```python
from build123d import *

# Parameters (mm, degrees)
BOSS_EXTRUDE1_DEPTH = 3.175
SKETCH2_W           = 25.4
SKETCH2_H           = 17.4625
BOSS_EXTRUDE2_DEPTH = 3.175
SKETCH4_W           = 2.238000096
SKETCH4_H           = 9.5
CUT_EXTRUDE1_DEPTH  = 3.175
SKETCH5_W           = 8.68426
SKETCH5_H           = 7.9625
BOSS_EXTRUDE3_DEPTH = 3.175
CUT_EXTRUDE2_DEPTH  = 3.175


with BuildPart() as part:
    # Sketch1 → Boss-Extrude1 (new body)
    with BuildSketch(Plane.XY):
        Polygon((-12.7, 19.05), (-6.35, 19.05), (-6.35, 15.875), (6.35, 15.875), (6.35, 19.05), (12.7, 19.05), (12.7, -19.05), (6.35, -19.05), (6.35, -15.875), (-6.35, -15.875), (-6.35, -19.05), (-12.7, -19.05), align=None)
    extrude(amount=BOSS_EXTRUDE1_DEPTH)

    # Sketch2 → Boss-Extrude2 (add)
    with BuildSketch(Plane(origin=(0, 0, 0), x_dir=(-1, 0, 0), z_dir=(0, 0, -1))):
        with Locations((0, -27.78125)):
            Rectangle(SKETCH2_W, SKETCH2_H)
    extrude(amount=-BOSS_EXTRUDE2_DEPTH)

    # Sketch4 → Cut-Extrude1 (cut)
    with BuildSketch(Plane(origin=(0, 0, 0), x_dir=(-1, 0, 0), z_dir=(0, 0, -1))):
        with Locations((-11.580999952, -23.8)):
            Rectangle(SKETCH4_W, SKETCH4_H)
    cut_extrude1 = extrude(amount=-CUT_EXTRUDE1_DEPTH, mode=Mode.SUBTRACT)

    # Sketch5 → Boss-Extrude3 (add)
    with BuildSketch(Plane(origin=(0, 0, 0), x_dir=(-1, 0, 0), z_dir=(0, 0, -1))):
        with Locations((-17.04213, -32.53125)):
            Rectangle(SKETCH5_W, SKETCH5_H)
    boss_extrude3 = extrude(amount=-BOSS_EXTRUDE3_DEPTH)

    # Sketch6 → Cut-Extrude2 (cut)
    with BuildSketch(Plane(origin=(0, 0, 0), x_dir=(-1, 0, 0), z_dir=(0, 0, -1))):
        Polygon((-21.38426, -33.3375), (-15.03426, -36.5125), (-21.38426, -36.5125), align=None)
    cut_extrude2 = extrude(amount=-CUT_EXTRUDE2_DEPTH, mode=Mode.SUBTRACT)

    # Mirror1: Cut-Extrude1, Boss-Extrude3, Cut-Extrude2 across plane
    add(cut_extrude1.mirror(Plane(origin=(0, 0, 0), x_dir=(0, 0, 1), z_dir=(1, 0, 0))), mode=Mode.SUBTRACT)
    add(boss_extrude3.mirror(Plane(origin=(0, 0, 0), x_dir=(0, 0, 1), z_dir=(1, 0, 0))))
    add(cut_extrude2.mirror(Plane(origin=(0, 0, 0), x_dir=(0, 0, 1), z_dir=(1, 0, 0))), mode=Mode.SUBTRACT)


solid = part.part
```
Check sheet for the modelled part. Datum: model origin and axes. Units: mm. A direction names the side the tool comes from. Round coordinates to 2 decimals unless told otherwise and drop trailing zeros. Order: outer loops, then holes, each group sorted by start corner. A loop starts at its lowest first (then second) coordinate and runs counter-clockwise, first axis right, second up.
1) Tool access check on faces 1 (the flat face through (-12.7, 0, 2)), 2 (the flat face through (-12, -19.05, 2)), 3 (the flat face through (12.7, 0, 2)). Record the directions out of +Z, -Z, +X, -X, +Y, -Y that give a thin tool (end or side, any length) a straight path to the whole face; none if there is none.
2) Section check D-D (y = 3.5). Record the boundary of the cut face in (x, z) (3 decimals), and give its area (3 significant figures).
3) Mould release check, pull along Y, two halves, no side actions. Record for faces 4 (the flat face through (0, -15.875, 2)), 5 (the flat face through (18.254, -34.903, 1.565)), 6 (the flat face through (6.35, 17, 2)), 7 (the flat face through (10.462, -24, 2)): +Y half, -Y half, draft (parallel to the pull), parting line (faces both ways), or undercut.
4) Go/stop test with flat-tipped pins: pin 1 Ø1 at (y, z) = (-23.5, 2) entering from +X; pin 2 Ø1.6 at (y, z) = (-23, 1.5) entering from -X; pin 3 Ø1 at (y, z) = (-3, 2) entering from +X. Record where each tip stops, or that it passes through.
5) Scan lines: line 1 (Y direction, x = -12.5, z = 2.7); line 2 (X direction, y = -18, z = 3); line 3 (X direction, y = -24, z = 0.2). Record each from-to range of solid material in increasing order.
Result:
1. face 1: +Z, -Z, -X, +Y
1. face 2: +Z, -Z, -X
1. face 3: +Z, -Z, +X, +Y
2. outline: (-12.7, 0) - (12.7, 0) - (12.7, 3.175) - (-12.7, 3.175) - close
2. area: 80.6 mm2
3. face 4: undercut
3. face 5: -Y half
3. face 6: draft
3. face 7: undercut
4. pin 1: stops at x = 10.46
4. pin 2: stops at x = -10.46
4. pin 3: stops at x = 12.7
5. line 1: y = -36.51 to -28.55, -19.05 to 19.05
5. line 2: x = -12.7 to -6.35, 6.35 to 12.7
5. line 3: x = -10.46 to 10.46
